```python
from build123d import *

# Parameters (mm, degrees)
BOSS_EXTRUDE1_DEPTH = 254
SKETCH2_R           = 152.4
CUT_EXTRUDE1_DEPTH  = 2033


with BuildPart() as part:
    # Sketch1 → Boss-Extrude1 (new body, symmetric)
    with BuildSketch(Plane.XY):
        with BuildLine():
            Line((-304.8, 2032), (304.8, 2032))
            Line((304.8, 2032), (304.8, 1845.579381215))
            ThreePointArc((304.8, 1845.579381215), (321.395341304, 1789.930769373), (365.76, 1752.461443094))
            ThreePointArc((365.76, 1752.461443094), (739.043152086, 1452.863164343), (909.828, 1005.725628473))
            ThreePointArc((909.828, 1005.725628473), (944.665425516, 938.847656099), (1016, 914.4))
            Line((1016, 914.4), (1016, 0))
            Line((1016, 0), (609.6, 0))
            Line((609.6, 0), (609.6, 304.8))
            Line((609.6, 304.8), (762, 304.8))
            Line((762, 304.8), (762, 914.4))
            Line((762, 914.4), (609.6, 914.4))
            ThreePointArc((609.6, 914.4), (0, 1524), (-609.6, 914.4))
            Line((-609.6, 914.4), (-762, 914.4))
            Line((-762, 914.4), (-762, 304.8))
            Line((-762, 304.8), (-609.6, 304.8))
            Line((-609.6, 304.8), (-609.6, 0))
            Line((-609.6, 0), (-1016, 0))
            Line((-1016, 0), (-1016, 914.4))
            ThreePointArc((-1016, 914.4), (-944.665425516, 938.847656099), (-909.828, 1005.725628473))
            ThreePointArc((-909.828, 1005.725628473), (-739.043152086, 1452.863164343), (-365.76, 1752.461443094))
            ThreePointArc((-365.76, 1752.461443094), (-321.395341304, 1789.930769373), (-304.8, 1845.579381215))
            Line((-304.8, 1845.579381215), (-304.8, 2032))
        make_face()
    extrude(amount=BOSS_EXTRUDE1_DEPTH, both=True)

    # Sketch2 → Cut-Extrude1 (cut, through all)
    with BuildSketch(Plane(origin=(0, 2032, 0), x_dir=(1, 0, 0), z_dir=(0, 1, 0))):
        Circle(SKETCH2_R)
    extrude(amount=-CUT_EXTRUDE1_DEPTH, mode=Mode.SUBTRACT)


solid = part.part
```
For this review, take the finished solid that the model builds, in its own axes (mm). A direction names the side the tool comes from. Give positions to 0.01 mm unless a question says otherwise; leave off trailing zeros. Order: outer loops, then holes, each group sorted by start corner. A loop starts at its lowest first (then second) coordinate and runs counter-clockwise, first axis right, second up.
1) Wall thickness on line 1 (Z direction, x = 0, y = 1776); line 2 (X direction, y = 360.5, z = 210); line 3 (X direction, y = 1250, z = -213.5): over which ranges is each line inside the solid? List them lowest first.
2) Take a section at C-C (z = 0). Give the boundary of the cut face in (x, y), then the cut area to 3 significant figures.
3) The part is to be moulded in two halves that separate along X. For faces 4 (the face through (-304.8, 1937, 4)), 5 (the face through (1016, 464, 4)), 6 (the face through (-762, 614, 4)), say which applies: released by +X, released by -X, zero draft, split by the parting line, or undercut.
4) For faces 1 (the face through (-609.6, 155, 4)), 2 (the face through (816, 0, 4)), 3 (the face through (685, 304.8, 4)), list the 3-axis set-ups (+Z, -Z, +X, -X, +Y, -Y) from which the entire face can be reached by the end or side of a thin tool; tool diameter is ignored.
5) Take a section at A-A (y = 485). Give the boundary of the cut face in (x, z).
6) Take a section at B-B (x = 0). Give the boundary of the cut face in (y, z).
7) Take a section at D-D (z = -216.5). Give the boundary of the cut face in (x, y).
8) Insertion check: pin 1 (2 mm diameter, centred on x = -321, z = -93, fed in from -Y); pin 2 (1 mm diameter, centred on y = 1200, z = 61.5, fed in from -X); pin 3 (10 mm diameter, centred on x = -254, z = -88, fed in from -Y). Each pin has a flat end and moves straight along its axis. Give the tip position at first contact, or say it passes through.
Derived:
1. line 1: z = -254 to -152.4, 152.4 to 254
1. line 2: x = -1016 to -762, 762 to 1016
1. line 3: x = -850.59 to -508.91, 508.91 to 850.59
2. outline: (-1016, 0) - (-609.6, 0) - (-609.6, 304.8) - (-762, 304.8) - (-762, 914.4) - (-609.6, 914.4) arc R609.6 cw to (-152.4, 1504.64) - (-152.4, 2032) - (-304.8, 2032) - (-304.8, 1845.58) arc R101.6 cw to (-365.76, 1752.46) arc R914.4 ccw to (-909.83, 1005.73) arc R101.6 cw to (-1016, 914.4) - close; (152.4, 1504.64) arc R609.6 cw to (609.6, 914.4) - (762, 914.4) - (762, 304.8) - (609.6, 304.8) - (609.6, 0) - (1016, 0) - (1016, 914.4) arc R101.6 cw to (909.83, 1005.73) arc R914.4 ccw to (365.76, 1752.46) arc R101.6 cw to (304.8, 1845.58) - (304.8, 2032) - (152.4, 2032) - close
2. area: 1,270,000 mm2
3. face 4: released by -X
3. face 5: released by +X
3. face 6: undercut
4. face 1: +Z, -Z, -Y
4. face 2: +Z, -Z, +X, -X, -Y
4. face 3: +Z, -Z
5. outline: (-1016, -254) - (-762, -254) - (-762, 254) - (-1016, 254) - close; (762, -254) - (1016, -254) - (1016, 254) - (762, 254) - close
6. outline: (1524, -254) - (2032, -254) - (2032, -152.4) - (1524, -152.4) - close; (1524, 152.4) - (2032, 152.4) - (2032, 254) - (1524, 254) - close
7. outline: (-1016, 0) - (-609.6, 0) - (-609.6, 304.8) - (-762, 304.8) - (-762, 914.4) - (-609.6, 914.4) arc R609.6 cw to (609.6, 914.4) - (762, 914.4) - (762, 304.8) - (609.6, 304.8) - (609.6, 0) - (1016, 0) - (1016, 914.4) arc R101.6 cw to (909.83, 1005.73) arc R914.4 ccw to (365.76, 1752.46) arc R101.6 cw to (304.8, 1845.58) - (304.8, 2032) - (-304.8, 2032) - (-304.8, 1845.58) arc R101.6 cw to (-365.76, 1752.46) arc R914.4 ccw to (-909.83, 1005.73) arc R101.6 cw to (-1016, 914.4) - close
8. pin 1: stops at y = 1432.02
8. pin 2: stops at x = -868.82
8. pin 3: stops at y = 1466.24
